The listing builds one solid part. Answer for the finished solid, in the listing's coordinates (mm). Coordinates: 2 decimals unless noted, no trailing zeros. Loops run counter-clockwise (first coordinate to the right, second up) from the corner with the lowest first, then second, coordinate; pieces in that order, holes last. Notation, with made-up numbers: M 34.25,49.25 L 71.25,49.25 A35 ccw 71.25,88.25 Z; hole C -9,17 d4. An arc over 180 degrees is marked long. Return JSON: item names as keys, results as strings. Group by question number.
1. Section C-C (y = 0.9) is taken. Write down the section's boundary in (x, z).
2. Given P1, Ø0.5, axis at y = 4.5, z = -1.5, coming from the -X side; P2, Ø0.5, axis at x = 2, z = -3.5, coming from the +Y side, each flat-ended and moving along its own axis, determine where each tip first touches the part or whether it passes through.
3. Section B-B (z = -6) is taken. Write down the section's boundary in (x, y).
4. Section A-A (z = 46) is taken. Write down the section's boundary in (x, y).
5. Straight lines are drawn through the part: L1, parallel to X at y = 1.95, z = 46; L2, parallel to X at y = 3.7, z = -42.5; L3, parallel to Z at x = 1, y = 3.1. For each, find the intervals that lie inside material, in ascending order. Write a range as from..to.
```python
from build123d import *

# Parameters (mm, degrees)
SKETCH1_W      = 8
SKETCH1_H      = 100
EXTRUDE1_DEPTH = 5
SKETCH2_R      = 1.55
EXTRUDE4_DEPTH = 5
SKETCH4_R      = 1.55
EXTRUDE6_DEPTH = 5
SKETCH5_W      = 4
SKETCH5_H      = 70
EXTRUDE7_DEPTH = 5
SKETCH6_W      = 1.530516358
SKETCH6_H      = 21.618543552
EXTRUDE8_DEPTH = 1


with BuildPart() as part:
    # Sketch1 → Extrude1 (new body)
    with BuildSketch(Plane(origin=(0, 0, 0), x_dir=(1, 0, 0), z_dir=(0, 1, 0))):
        Rectangle(SKETCH1_W, SKETCH1_H)
    extrude(amount=EXTRUDE1_DEPTH)

    # Sketch2 → Extrude4 (cut)
    with BuildSketch(Plane(origin=(0, 5, 0), x_dir=(1, 0, 0), z_dir=(0, 1, 0))):
        with Locations(Location((0, -46, 0), (0, 0, 270))):
            Circle(SKETCH2_R)
    extrude(amount=-EXTRUDE4_DEPTH, mode=Mode.SUBTRACT)

    # Sketch4 → Extrude6 (cut)
    with BuildSketch(Plane(origin=(0, 5, 0), x_dir=(1, 0, 0), z_dir=(0, 1, 0))):
        with Locations((0, -43.46)):
            Circle(SKETCH4_R)
        with Locations((0, -46)):
            Circle(SKETCH4_R)
        with Locations(Location((-1, 42.5, 0), (0, 0, 270))):
            Circle(SKETCH4_R)
        with Locations(Location((0, 46, 0), (0, 0, 270))):
            Circle(SKETCH4_R)
    extrude(amount=-EXTRUDE6_DEPTH, mode=Mode.SUBTRACT)

    # Sketch5 → Extrude7 (cut)
    with BuildSketch(Plane(origin=(0, 5, 0), x_dir=(1, 0, 0), z_dir=(0, 1, 0))):
        with Locations((-2, 0)):
            Rectangle(SKETCH5_W, SKETCH5_H)
    extrude(amount=-EXTRUDE7_DEPTH, mode=Mode.SUBTRACT)

    # Sketch6 → Extrude8 (cut)
    with BuildSketch(Plane(origin=(0, 5, 0), x_dir=(1, 0, 0), z_dir=(0, 1, 0))):
        with Locations((2.112618746, 5.201364346)):
            Rectangle(SKETCH6_W, SKETCH6_H)
    extrude(amount=-EXTRUDE8_DEPTH, mode=Mode.SUBTRACT)


solid = part.part
```
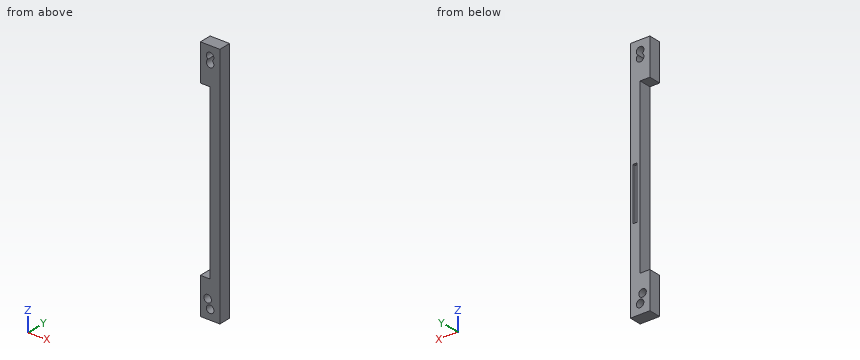
Worked out:
{
 "1": {"outline": "M -4,-50 L 4,-50 L 4,50 L -4,50 L -4,35 L 0,35 L 0,-35 L -4,-35 Z; hole C -1,-42.5 d3.1; hole C 0,-46 d3.1; hole M -0.89,44.73 A1.55 ccw long 0.89,44.73 A1.55 ccw long Z"},
 "2": {"P1": "x = 0", "P2": "y = 4"},
 "3": {"outline": "M 0,0 L 4,0 L 4,5 L 2.88,5 L 2.88,4 L 1.35,4 L 1.35,5 L 0,5 Z"},
 "4": {"outline": "M -4,0 L -1.55,0 L -1.55,5 L -4,5 Z; M 1.55,0 L 4,0 L 4,5 L 1.55,5 Z"},
 "5": {"L1": "-4..-1.55, 1.55..4", "L2": "-4..-2.55, 0.55..4", "L3": "-50..-47.18, -44.82..42.28, 44.64..44.82, 47.18..50"}
}
